Verification items for the finished model (mm, model axes). Face numbers are marked on the shaded views. Round coordinates to 2 decimals unless told otherwise and drop trailing zeros. Write each loop counter-clockwise with the first axis right and the second up, starting at its lowest first coordinate (ties: lowest second). Pieces come first, ordered by that corner, then holes. Notation, with made-up numbers: M 84,75 L 113,75 A18 ccw 113,108 Z; hole C 76.5,76.25 d11. An arc over 180 degrees is marked long. One line per question, with ' | ' between items.
from build123d import *

# Parameters (mm, degrees)
CHAMFER1_SIZE = 0.2


with BuildPart() as part:
    # Sketch1 → Revolve1 (revolve)
    with BuildSketch(Plane.XY, mode=Mode.PRIVATE) as revolve1_sk:
        Polygon((16.5, 0), (18.5, 0), (18.5, 4), (18.5, 56), (18.5, 60), (16.5, 60), (16.5, 56), (16.5, 4), align=None)
    revolve(revolve1_sk.sketch.rotate(Axis((0, 0, 0), (0, 1, 0)), 90), axis=Axis((0, 0, 0), (0, 1, 0)))

    # Chamfer1
    chamfer1_edges = [part.edges().sort_by_distance(p)[0] for p in [
        (0, 0, 16.5),
        (0, 60, 16.5),
        (0, 60, 18.5),
        (0, 0, 18.5),
    ]]
    chamfer(chamfer1_edges, length=CHAMFER1_SIZE)


solid = part.part
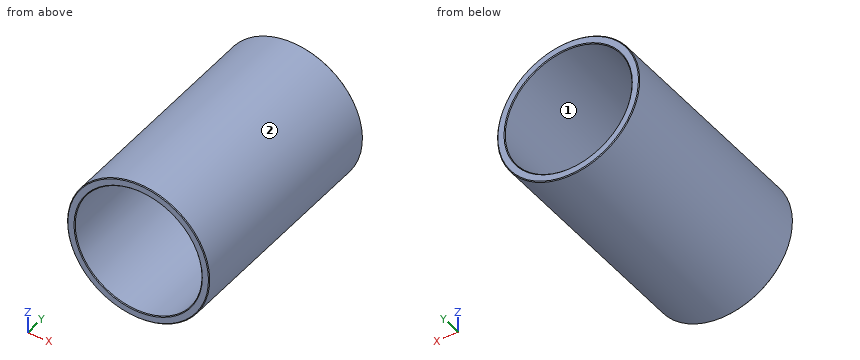
1. Section check A-A, the plane x = 0. Record the cut outline in (y, z), then the cut area to 3 significant figures.
Results:
outline: M 0,-18.3 L 0.2,-18.5 L 59.8,-18.5 L 60,-18.3 L 60,-16.7 L 59.8,-16.5 L 0.2,-16.5 L 0,-16.7 Z; M 0,16.7 L 0.2,16.5 L 59.8,16.5 L 60,16.7 L 60,18.3 L 59.8,18.5 L 0.2,18.5 L 0,18.3 Z | area: 240 mm2
2. Go/stop test with flat-tipped pins: P1, Ø20, axis at x = 0, z = 0, coming from the -Y side; P2, Ø3, axis at y = 7.5, z = -8.5, coming from the +X side; P3, Ø4, axis at x = 10, y = 42.5, coming from the -Z side; P4, Ø1, axis at x = 13, y = 29, coming from the +Z side. Record where each tip stops, or that it passes through.
Results:
P1: passes through | P2: stops at x = 17.12 | P3: stops at z = -16.68 | P4: stops at z = 13.64
3. Section check B-B, the plane z = 0. Record the cut outline in (x, y), then the cut area to 3 significant figures.
Results:
outline: M -18.5,0.2 L -18.3,0 L -16.7,0 L -16.5,0.2 L -16.5,59.8 L -16.7,60 L -18.3,60 L -18.5,59.8 Z; M 16.5,0.2 L 16.7,0 L 18.3,0 L 18.5,0.2 L 18.5,59.8 L 18.3,60 L 16.7,60 L 16.5,59.8 Z | area: 240 mm2
4. Mould release check, pull along Z, two halves, no side actions. Record for the marked faces 1 and 2: pulls with the +Z half, pulls with the -Z half, needs draft (parallel to the pull), parting line crosses it, or undercut.
Results:
face 1: undercut | face 2: parting line crosses it
5. Section check C-C, the plane y = 23. Record the cut outline in (x, z), then the cut area to 3 significant figures.
Results:
outline: C 0,0 d37; hole C 0,0 d33 | area: 220 mm2
6. Thickness scan on line 1 (X direction, y = 25, z = 0); line 2 (X direction, y = 11.5, z = 9); line 3 (Z direction, x = -7, y = 23.5). Record the ranges inside material, lowest first.
Results:
line 1: x = -18.5 to -16.5, 16.5 to 18.5 | line 2: x = -16.16 to -13.83, 13.83 to 16.16 | line 3: z = -17.12 to -14.94, 14.94 to 17.12
